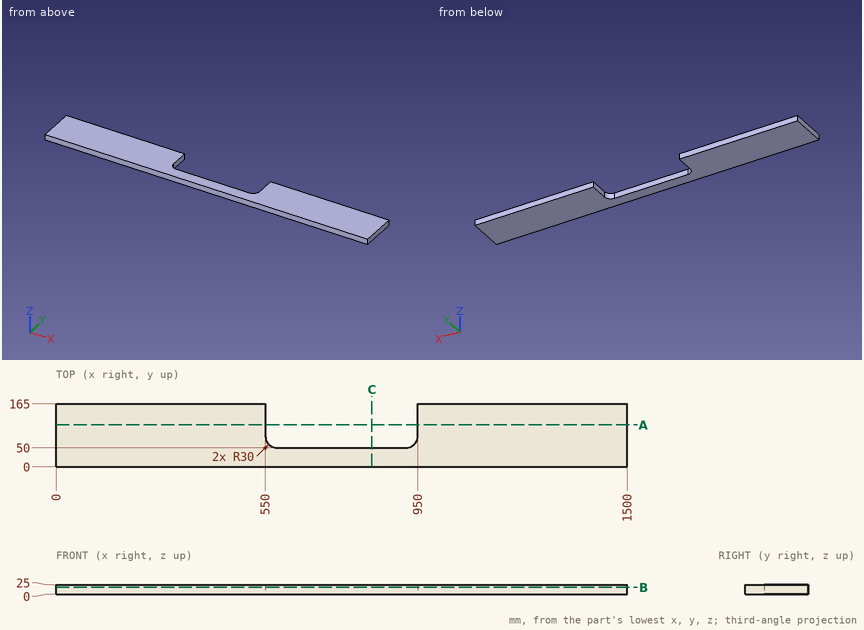
Drawing for the job (mm, zero at the part's lowest x, y, z). Round coordinates to 2 decimals unless told otherwise and drop trailing zeros. Loops run counter-clockwise (first coordinate to the right, second up) from the corner with the lowest first, then second, coordinate; pieces in that order, holes last. Notation, with made-up numbers: (-26, 22.25) -> (14, 22.25) arc R22 ccw to (14, 53.25) -> close; hole circle Ø4 at (49, -14.5). An arc over 180 degrees is marked (long way). Answer as CSV lines item,"result". Start each with the question number.
1) Slice it at B-B (z = 18.5). List the corners of the cut face in (x, y), plus the area to 3 significant figures.
2) Slice it at A-A (y = 110). List the corners of the cut face in (x, z), plus the area to 3 significant figures.
3) Slice it at C-C (x = 829.5). List the corners of the cut face in (y, z).
4) Pin check, flat tip, straight feed: P1, Ø12.5, axis at x = 674.5, z = 7, coming from the +Y side. Stop position of the tip, or through.
5) Probe line 1 along X through (y, z) = (105.5, 12.75); line 2 along X through (y, z) = (77, 17); line 3 along Y through (x, z) = (675, 8.75). List the from-to ranges inside material, lowest first.
Filled in:
1,outline,"(0, 0) -> (1500, 0) -> (1500, 165) -> (950, 165) -> (950, 80) arc R30 cw to (920, 50) -> (580, 50) arc R30 cw to (550, 80) -> (550, 165) -> (0, 165) -> close"
1,area,"202,000 mm2"
2,outline,"(0, 0) -> (550, 0) -> (550, 25) -> (0, 25) -> close; (950, 0) -> (1500, 0) -> (1500, 25) -> (950, 25) -> close"
2,area,"27,500 mm2"
3,outline,"(0, 0) -> (50, 0) -> (50, 25) -> (0, 25) -> close"
4,P1,"stops at y = 50"
5,line 1,"x = 0 to 550, 950 to 1500"
5,line 2,"x = 0 to 550.15, 949.85 to 1500"
5,line 3,"y = 0 to 50"
